CAD build for the part. Positions are in the model's coordinates, mm. A direction names the side the tool comes from. Round coordinates to 2 decimals unless told otherwise and drop trailing zeros. Order: outer loops, then holes, each group sorted by start corner. A loop starts at its lowest first (then second) coordinate and runs counter-clockwise, first axis right, second up. Notation, with made-up numbers: (23, 6.5) - (27, 6.5) arc R6 cw to (27, 16.5) - close; hole circle Ø1 at (10.25, 15.5). An arc over 180 degrees is marked (long way). Write item = value, one per line.
from build123d import *

# Parameters (mm, degrees)
SKETCH1_W      = 6.6675
SKETCH1_H      = 69.215
EXTRUDE1_DEPTH = 4.318
EXTRUDE2_DEPTH = 1.7653
EXTRUDE3_DEPTH = 5.969
SKETCH4_R      = 1.5875
EXTRUDE4_DEPTH = 71.131650408
SKETCH5_R      = 0.635
EXTRUDE5_DEPTH = 6.35


with BuildPart() as part:
    # Sketch1 → Extrude1 (new body)
    with BuildSketch(Plane(origin=(0, 0, 0), x_dir=(1, 0, 0), z_dir=(0, 1, 0))):
        with Locations((3.33375, 34.6075)):
            Rectangle(SKETCH1_W, SKETCH1_H)
    extrude(amount=EXTRUDE1_DEPTH)

    # Sketch2 → Extrude2 (add)
    with BuildSketch(Plane(origin=(0, 4.318, 0), x_dir=(1, 0, 0), z_dir=(0, 1, 0))):
        with BuildLine():
            Line((-1.5875, 69.215), (8.255, 69.215))
            ThreePointArc((8.255, 69.215), (9.153025612, 68.843025612), (9.525, 67.945))
            Line((9.525, 67.945), (9.525, 1.27))
            ThreePointArc((9.525, 1.27), (9.153025612, 0.371974388), (8.255, 0))
            Line((8.255, 0), (-1.5875, 0))
            ThreePointArc((-1.5875, 0), (-2.485525612, 0.371974388), (-2.8575, 1.27))
            Line((-2.8575, 1.27), (-2.8575, 67.945))
            ThreePointArc((-2.8575, 67.945), (-2.485525612, 68.843025612), (-1.5875, 69.215))
        make_face()
    extrude(amount=EXTRUDE2_DEPTH)

    # Sketch3 → Extrude3 (add)
    with BuildSketch(Plane(origin=(0, 6.0833, 0), x_dir=(1, 0, 0), z_dir=(0, 1, 0))):
        with BuildLine():
            Line((-0.47625, 59.407898598), (-0.47625, 9.172101402))
            ThreePointArc((-0.47625, 9.172101402), (-0.175285378, 8.351205284), (0.584963286, 7.919381119))
            Line((0.584963286, 7.919381119), (5.664963286, 7.072714452))
            ThreePointArc((5.664963286, 7.072714452), (6.694646118, 7.356399358), (7.14375, 8.325434736))
            Line((7.14375, 8.325434736), (7.14375, 60.254565264))
            ThreePointArc((7.14375, 60.254565264), (6.694646118, 61.223600642), (5.664963286, 61.507285548))
            Line((5.664963286, 61.507285548), (0.584963286, 60.660618881))
            ThreePointArc((0.584963286, 60.660618881), (-0.175285378, 60.228794716), (-0.47625, 59.407898598))
        make_face()
    extrude(amount=EXTRUDE3_DEPTH)

    # Sketch4 → Extrude4 (cut, through all)
    with BuildSketch(Plane(origin=(0, 6.0833, 0), x_dir=(1, 0, 0), z_dir=(0, 1, 0))):
        with Locations(Location((3.33375, 66.3575, 0), (0, 0, 270))):
            Circle(SKETCH4_R)
        with Locations(Location((3.33375, 2.8575, 0), (0, 0, 270))):
            Circle(SKETCH4_R)
    extrude(amount=-EXTRUDE4_DEPTH, mode=Mode.SUBTRACT)

    # Sketch5 → Extrude5 (cut)
    with BuildSketch(Plane(origin=(0, 12.0523, 0), x_dir=(1, 0, 0), z_dir=(0, 1, 0))):
        with Locations((5.11175, 57.15)):
            Circle(SKETCH5_R)
        with Locations((1.55575, 55.88)):
            Circle(SKETCH5_R)
        with Locations((5.11175, 54.61)):
            Circle(SKETCH5_R)
        with Locations((5.11175, 52.07)):
            Circle(SKETCH5_R)
        with Locations((5.11175, 49.53)):
            Circle(SKETCH5_R)
        with Locations((5.11175, 46.99)):
            Circle(SKETCH5_R)
        with Locations((5.11175, 44.45)):
            Circle(SKETCH5_R)
        with Locations((5.11175, 41.91)):
            Circle(SKETCH5_R)
        with Locations((5.11175, 39.37)):
            Circle(SKETCH5_R)
        with Locations((5.11175, 36.83)):
            Circle(SKETCH5_R)
        with Locations((5.11175, 34.29)):
            Circle(SKETCH5_R)
        with Locations((5.11175, 31.75)):
            Circle(SKETCH5_R)
        with Locations((5.11175, 29.21)):
            Circle(SKETCH5_R)
        with Locations((5.11175, 26.67)):
            Circle(SKETCH5_R)
        with Locations((5.11175, 24.13)):
            Circle(SKETCH5_R)
        with Locations((5.11175, 21.59)):
            Circle(SKETCH5_R)
        with Locations((5.11175, 19.05)):
            Circle(SKETCH5_R)
        with Locations((5.11175, 16.51)):
            Circle(SKETCH5_R)
        with Locations((5.11175, 13.97)):
            Circle(SKETCH5_R)
        with Locations((5.11175, 11.43)):
            Circle(SKETCH5_R)
        with Locations((1.55575, 53.34)):
            Circle(SKETCH5_R)
        with Locations((1.55575, 50.8)):
            Circle(SKETCH5_R)
        with Locations((1.55575, 48.26)):
            Circle(SKETCH5_R)
        with Locations((1.55575, 45.72)):
            Circle(SKETCH5_R)
        with Locations((1.55575, 43.18)):
            Circle(SKETCH5_R)
        with Locations((1.55575, 40.64)):
            Circle(SKETCH5_R)
        with Locations((1.55575, 38.1)):
            Circle(SKETCH5_R)
        with Locations((1.55575, 35.56)):
            Circle(SKETCH5_R)
        with Locations((1.55575, 33.02)):
            Circle(SKETCH5_R)
        with Locations((1.55575, 30.48)):
            Circle(SKETCH5_R)
        with Locations((1.55575, 27.94)):
            Circle(SKETCH5_R)
        with Locations((1.55575, 25.4)):
            Circle(SKETCH5_R)
        with Locations((1.55575, 22.86)):
            Circle(SKETCH5_R)
        with Locations((1.55575, 20.32)):
            Circle(SKETCH5_R)
        with Locations((1.55575, 17.78)):
            Circle(SKETCH5_R)
        with Locations((1.55575, 15.24)):
            Circle(SKETCH5_R)
        with Locations((1.55575, 12.7)):
            Circle(SKETCH5_R)
    extrude(amount=-EXTRUDE5_DEPTH, mode=Mode.SUBTRACT)


solid = part.part
(1) Pull direction Z, two halves, no side cores. Call faces 1 (the cylindrical face through (9.16, 5.19, -0.38)), 2 (the flat face through (2, 5.702, -56)), 3 (the flat face through (0, 2, -34)): released by +Z, released by -Z, zero draft, split by the parting line, or undercut.
Solved:
face_1 = released by +Z
face_2 = undercut
face_3 = zero draft
(2) Tool access for faces 4 (the flat face through (-0.476, 9, -35)), 5 (the cylindrical face through (2.7, 3.1, -64.9)), 6 (the flat face through (5, 5.702, -29)): list every direction of +Z, -Z, +X, -X, +Y, -Y with a clear straight run to the whole face (end or side of a thin tool).
Solved:
face_4 = +Z, -Z, -X, +Y
face_5 = +Y, -Y
face_6 = +Y
(3) Probe line 1 along Z through (x, y) = (4.5, 4.75) (3 decimals); line 2 along Y through (x, z) = (4, -63); line 3 along X through (y, z) = (8, -40.64). List the from-to ranges inside material, lowest first.
Solved:
line_1 = -69.215 to -67.435, -65.28 to -3.935, -1.78 to 0
line_2 = 0 to 6.08
line_3 = -0.48 to 0.92, 2.19 to 7.14
(4) Band-saw the part on A-A on z = -48.26. List the corners of the cut face in (x, y) (1 decimal), plus the area to 3 significant figures.
Solved:
outline = (-2.9, 4.3) - (0, 4.3) - (0, 0) - (6.7, 0) - (6.7, 4.3) - (9.5, 4.3) - (9.5, 6.1) - (7.1, 6.1) - (7.1, 12.1) - (2.2, 12.1) - (2.2, 5.7) - (0.9, 5.7) - (0.9, 12.1) - (-0.5, 12.1) - (-0.5, 6.1) - (-2.9, 6.1) - close
area = 88.1 mm²
(5) Drop flat-ended pins along their axis: pin 1 (0.6 mm diameter, centred on x = 5, z = -42, fed in from +Y); pin 2 (3 mm diameter, centred on y = 9, z = -41.5, fed in from +X); pin 3 (4.5 mm diameter, centred on y = 1, z = -43, fed in from +X). Give the stop position or say it passes through.
Solved:
pin_1 = 5.7
pin_2 = 7.14
pin_3 = 6.67
(6) Band-saw the part on B-B on y = 8.75. Count the separate pieces of the cut face and the enclosed holes in it, plus the area to 3 significant figures.
Solved:
separate_pieces = 1
enclosed_holes = 37
area = 361 mm²
